Work out the finished part from the listing and answer in its coordinate system (mm). A direction names the side the tool comes from. Give positions to 0.01 mm unless a question says otherwise; leave off trailing zeros. Loops run counter-clockwise (first coordinate to the right, second up) from the corner with the lowest first, then second, coordinate; pieces in that order, holes last.
from build123d import *

# Parameters (mm, degrees)
SKETCH1_W                  = 267
SKETCH1_H                  = 96
BOSS_EXTRUDE1_DEPTH        = 10
SKETCH5_W                  = 261
SKETCH5_H                  = 90
CUT_EXTRUDE2_DEPTH         = 1.7
SKETCH2_R                  = 9.25
CUT_EXTRUDE1_DEPTH         = 10
LPATTERN1_COUNT            = 4
LPATTERN1_PITCH            = 21.5
LPATTERN1_COUNT_DIR2       = 12
LPATTERN1_PITCH_DIR2       = 21.5
ADVANCEDHOLE2_OUTLINE_R    = 2.640558065
ADVANCEDHOLE2_DEPTH        = 7.996
ADVANCEDHOLE2_DRAFT        = -2.3593
ADVANCEDHOLE2_2_OUTLINE_R  = 2.640558065
ADVANCEDHOLE2_2_DEPTH      = 7.996
ADVANCEDHOLE2_2_DRAFT      = -2.3593
ADVANCEDHOLE2_3_OUTLINE_R  = 2.640558065
ADVANCEDHOLE2_3_DEPTH      = 7.996
ADVANCEDHOLE2_3_DRAFT      = -2.3593
ADVANCEDHOLE2_4_OUTLINE_R  = 2.640558065
ADVANCEDHOLE2_4_DEPTH      = 7.996
ADVANCEDHOLE2_4_DRAFT      = -2.3593
ADVANCEDHOLE2_5_OUTLINE_R  = 2.640558065
ADVANCEDHOLE2_5_DEPTH      = 7.996
ADVANCEDHOLE2_5_DRAFT      = -2.3593
ADVANCEDHOLE2_6_OUTLINE_R  = 2.640558065
ADVANCEDHOLE2_6_DEPTH      = 7.996
ADVANCEDHOLE2_6_DRAFT      = -2.3593
ADVANCEDHOLE2_7_OUTLINE_R  = 2.640558065
ADVANCEDHOLE2_7_DEPTH      = 7.996
ADVANCEDHOLE2_7_DRAFT      = -2.3593
ADVANCEDHOLE2_8_OUTLINE_R  = 2.640558065
ADVANCEDHOLE2_8_DEPTH      = 7.996
ADVANCEDHOLE2_8_DRAFT      = -2.3593
ADVANCEDHOLE2_9_OUTLINE_R  = 2.640558065
ADVANCEDHOLE2_9_DEPTH      = 7.996
ADVANCEDHOLE2_9_DRAFT      = -2.3593
ADVANCEDHOLE2_10_OUTLINE_R = 2.640558065
ADVANCEDHOLE2_10_DEPTH     = 7.996
ADVANCEDHOLE2_10_DRAFT     = -2.3593


# Read off the part's stored shape, not the designer's step: AdvancedHole2
with BuildPart() as part:
    # Sketch1 → Boss-Extrude1 (new body)
    with BuildSketch(Plane(origin=(0, 0, 0), x_dir=(1, 0, 0), z_dir=(0, 1, 0))):
        with Locations((133.5, 48)):
            Rectangle(SKETCH1_W, SKETCH1_H)
    extrude(amount=BOSS_EXTRUDE1_DEPTH)

    # Sketch5 → Cut-Extrude2 (cut)
    with BuildSketch(Plane(origin=(0, 10, 0), x_dir=(1, 0, 0), z_dir=(0, 1, 0))):
        with Locations((133.5, 48)):
            Rectangle(SKETCH5_W, SKETCH5_H)
    extrude(amount=-CUT_EXTRUDE2_DEPTH, mode=Mode.SUBTRACT)

    # Sketch2 → Cut-Extrude1 (cut)
    with BuildSketch(Plane(origin=(0, 10, 0), x_dir=(1, 0, 0), z_dir=(0, 1, 0))):
        with Locations(Location((15.25, 15.75, 0), (0, 0, 270))):
            Circle(SKETCH2_R)
    cut_extrude1 = extrude(amount=-CUT_EXTRUDE1_DEPTH, mode=Mode.SUBTRACT)

    # LPattern1: Cut-Extrude1 4 × 12
    with Locations(*[(j * LPATTERN1_PITCH_DIR2, 0, -i * LPATTERN1_PITCH) for i in range(LPATTERN1_COUNT) for j in range(LPATTERN1_COUNT_DIR2) if (i, j) != (0, 0)]):
        add(cut_extrude1, mode=Mode.SUBTRACT)


with BuildPart() as advancedhole2_tool:
    # AdvancedHole2 outline → AdvancedHole2 (with draft: the straight prism first)
    with BuildSketch(Plane(origin=(0, 0.304, 0), x_dir=(1, 0, 0), z_dir=(0, 1, 0))):
        with Locations((155, 69.5)):
            Circle(ADVANCEDHOLE2_OUTLINE_R)
    extrude(amount=ADVANCEDHOLE2_DEPTH)
    # AdvancedHole2: the draft: its side faces are tilted about the plane it starts from
    advancedhole2_sides = [advancedhole2_tool.faces().sort_by_distance(p)[0] for p in [
        (152.359441935, 4.302, -69.5),
    ]]
    draft(advancedhole2_sides, Plane(origin=(0, 0.304, 0), x_dir=(1, 0, 0), z_dir=(0, 1, 0)), ADVANCEDHOLE2_DRAFT)


with BuildPart() as part_1:
    add(part.part)

    # AdvancedHole2: cut by advancedhole2_tool
    add(advancedhole2_tool.part, mode=Mode.SUBTRACT)


with BuildPart() as advancedhole2_2_tool:
    # AdvancedHole2 2 outline → AdvancedHole2 2 (with draft: the straight prism first)
    with BuildSketch(Plane(origin=(0, 0.304, 0), x_dir=(1, 0, 0), z_dir=(0, 1, 0))):
        with Locations((155, 26.5)):
            Circle(ADVANCEDHOLE2_2_OUTLINE_R)
    extrude(amount=ADVANCEDHOLE2_2_DEPTH)
    # AdvancedHole2 2: the draft: its side faces are tilted about the plane it starts from
    advancedhole2_2_sides = [advancedhole2_2_tool.faces().sort_by_distance(p)[0] for p in [
        (152.359441935, 4.302, -26.5),
    ]]
    draft(advancedhole2_2_sides, Plane(origin=(0, 0.304, 0), x_dir=(1, 0, 0), z_dir=(0, 1, 0)), ADVANCEDHOLE2_2_DRAFT)


with BuildPart() as part_2:
    add(part_1.part)

    # AdvancedHole2 2: cut by advancedhole2_2_tool
    add(advancedhole2_2_tool.part, mode=Mode.SUBTRACT)


with BuildPart() as advancedhole2_3_tool:
    # AdvancedHole2 3 outline → AdvancedHole2 3 (with draft: the straight prism first)
    with BuildSketch(Plane(origin=(0, 0.304, 0), x_dir=(1, 0, 0), z_dir=(0, 1, 0))):
        with Locations((112, 26.5)):
            Circle(ADVANCEDHOLE2_3_OUTLINE_R)
    extrude(amount=ADVANCEDHOLE2_3_DEPTH)
    # AdvancedHole2 3: the draft: its side faces are tilted about the plane it starts from
    advancedhole2_3_sides = [advancedhole2_3_tool.faces().sort_by_distance(p)[0] for p in [
        (109.359441935, 4.302, -26.5),
    ]]
    draft(advancedhole2_3_sides, Plane(origin=(0, 0.304, 0), x_dir=(1, 0, 0), z_dir=(0, 1, 0)), ADVANCEDHOLE2_3_DRAFT)


with BuildPart() as part_3:
    add(part_2.part)

    # AdvancedHole2 3: cut by advancedhole2_3_tool
    add(advancedhole2_3_tool.part, mode=Mode.SUBTRACT)


with BuildPart() as advancedhole2_4_tool:
    # AdvancedHole2 4 outline → AdvancedHole2 4 (with draft: the straight prism first)
    with BuildSketch(Plane(origin=(0, 0.304, 0), x_dir=(1, 0, 0), z_dir=(0, 1, 0))):
        with Locations((112, 69.5)):
            Circle(ADVANCEDHOLE2_4_OUTLINE_R)
    extrude(amount=ADVANCEDHOLE2_4_DEPTH)
    # AdvancedHole2 4: the draft: its side faces are tilted about the plane it starts from
    advancedhole2_4_sides = [advancedhole2_4_tool.faces().sort_by_distance(p)[0] for p in [
        (109.359441935, 4.302, -69.5),
    ]]
    draft(advancedhole2_4_sides, Plane(origin=(0, 0.304, 0), x_dir=(1, 0, 0), z_dir=(0, 1, 0)), ADVANCEDHOLE2_4_DRAFT)


with BuildPart() as part_4:
    add(part_3.part)

    # AdvancedHole2 4: cut by advancedhole2_4_tool
    add(advancedhole2_4_tool.part, mode=Mode.SUBTRACT)


with BuildPart() as advancedhole2_5_tool:
    # AdvancedHole2 5 outline → AdvancedHole2 5 (with draft: the straight prism first)
    with BuildSketch(Plane(origin=(0, 0.304, 0), x_dir=(1, 0, 0), z_dir=(0, 1, 0))):
        with Locations((198, 48)):
            Circle(ADVANCEDHOLE2_5_OUTLINE_R)
    extrude(amount=ADVANCEDHOLE2_5_DEPTH)
    # AdvancedHole2 5: the draft: its side faces are tilted about the plane it starts from
    advancedhole2_5_sides = [advancedhole2_5_tool.faces().sort_by_distance(p)[0] for p in [
        (195.359441935, 4.302, -48),
    ]]
    draft(advancedhole2_5_sides, Plane(origin=(0, 0.304, 0), x_dir=(1, 0, 0), z_dir=(0, 1, 0)), ADVANCEDHOLE2_5_DRAFT)


with BuildPart() as part_5:
    add(part_4.part)

    # AdvancedHole2 5: cut by advancedhole2_5_tool
    add(advancedhole2_5_tool.part, mode=Mode.SUBTRACT)


with BuildPart() as advancedhole2_6_tool:
    # AdvancedHole2 6 outline → AdvancedHole2 6 (with draft: the straight prism first)
    with BuildSketch(Plane(origin=(0, 0.304, 0), x_dir=(1, 0, 0), z_dir=(0, 1, 0))):
        with Locations((69, 48)):
            Circle(ADVANCEDHOLE2_6_OUTLINE_R)
    extrude(amount=ADVANCEDHOLE2_6_DEPTH)
    # AdvancedHole2 6: the draft: its side faces are tilted about the plane it starts from
    advancedhole2_6_sides = [advancedhole2_6_tool.faces().sort_by_distance(p)[0] for p in [
        (66.359441935, 4.302, -48),
    ]]
    draft(advancedhole2_6_sides, Plane(origin=(0, 0.304, 0), x_dir=(1, 0, 0), z_dir=(0, 1, 0)), ADVANCEDHOLE2_6_DRAFT)


with BuildPart() as part_6:
    add(part_5.part)

    # AdvancedHole2 6: cut by advancedhole2_6_tool
    add(advancedhole2_6_tool.part, mode=Mode.SUBTRACT)


with BuildPart() as advancedhole2_7_tool:
    # AdvancedHole2 7 outline → AdvancedHole2 7 (with draft: the straight prism first)
    with BuildSketch(Plane(origin=(0, 0.304, 0), x_dir=(1, 0, 0), z_dir=(0, 1, 0))):
        with Locations((26, 26.5)):
            Circle(ADVANCEDHOLE2_7_OUTLINE_R)
    extrude(amount=ADVANCEDHOLE2_7_DEPTH)
    # AdvancedHole2 7: the draft: its side faces are tilted about the plane it starts from
    advancedhole2_7_sides = [advancedhole2_7_tool.faces().sort_by_distance(p)[0] for p in [
        (23.359441935, 4.302, -26.5),
    ]]
    draft(advancedhole2_7_sides, Plane(origin=(0, 0.304, 0), x_dir=(1, 0, 0), z_dir=(0, 1, 0)), ADVANCEDHOLE2_7_DRAFT)


with BuildPart() as part_7:
    add(part_6.part)

    # AdvancedHole2 7: cut by advancedhole2_7_tool
    add(advancedhole2_7_tool.part, mode=Mode.SUBTRACT)


with BuildPart() as advancedhole2_8_tool:
    # AdvancedHole2 8 outline → AdvancedHole2 8 (with draft: the straight prism first)
    with BuildSketch(Plane(origin=(0, 0.304, 0), x_dir=(1, 0, 0), z_dir=(0, 1, 0))):
        with Locations((241, 26.5)):
            Circle(ADVANCEDHOLE2_8_OUTLINE_R)
    extrude(amount=ADVANCEDHOLE2_8_DEPTH)
    # AdvancedHole2 8: the draft: its side faces are tilted about the plane it starts from
    advancedhole2_8_sides = [advancedhole2_8_tool.faces().sort_by_distance(p)[0] for p in [
        (238.359441935, 4.302, -26.5),
    ]]
    draft(advancedhole2_8_sides, Plane(origin=(0, 0.304, 0), x_dir=(1, 0, 0), z_dir=(0, 1, 0)), ADVANCEDHOLE2_8_DRAFT)


with BuildPart() as part_8:
    add(part_7.part)

    # AdvancedHole2 8: cut by advancedhole2_8_tool
    add(advancedhole2_8_tool.part, mode=Mode.SUBTRACT)


with BuildPart() as advancedhole2_9_tool:
    # AdvancedHole2 9 outline → AdvancedHole2 9 (with draft: the straight prism first)
    with BuildSketch(Plane(origin=(0, 0.304, 0), x_dir=(1, 0, 0), z_dir=(0, 1, 0))):
        with Locations((241, 69.5)):
            Circle(ADVANCEDHOLE2_9_OUTLINE_R)
    extrude(amount=ADVANCEDHOLE2_9_DEPTH)
    # AdvancedHole2 9: the draft: its side faces are tilted about the plane it starts from
    advancedhole2_9_sides = [advancedhole2_9_tool.faces().sort_by_distance(p)[0] for p in [
        (238.359441935, 4.302, -69.5),
    ]]
    draft(advancedhole2_9_sides, Plane(origin=(0, 0.304, 0), x_dir=(1, 0, 0), z_dir=(0, 1, 0)), ADVANCEDHOLE2_9_DRAFT)


with BuildPart() as part_9:
    add(part_8.part)

    # AdvancedHole2 9: cut by advancedhole2_9_tool
    add(advancedhole2_9_tool.part, mode=Mode.SUBTRACT)


with BuildPart() as advancedhole2_10_tool:
    # AdvancedHole2 10 outline → AdvancedHole2 10 (with draft: the straight prism first)
    with BuildSketch(Plane(origin=(0, 0.304, 0), x_dir=(1, 0, 0), z_dir=(0, 1, 0))):
        with Locations((26, 69.5)):
            Circle(ADVANCEDHOLE2_10_OUTLINE_R)
    extrude(amount=ADVANCEDHOLE2_10_DEPTH)
    # AdvancedHole2 10: the draft: its side faces are tilted about the plane it starts from
    advancedhole2_10_sides = [advancedhole2_10_tool.faces().sort_by_distance(p)[0] for p in [
        (23.359441935, 4.302, -69.5),
    ]]
    draft(advancedhole2_10_sides, Plane(origin=(0, 0.304, 0), x_dir=(1, 0, 0), z_dir=(0, 1, 0)), ADVANCEDHOLE2_10_DRAFT)


with BuildPart() as part_10:
    add(part_9.part)

    # AdvancedHole2 10: cut by advancedhole2_10_tool
    add(advancedhole2_10_tool.part, mode=Mode.SUBTRACT)


solid = part_10.part
Item 1: Flat-ended cylindrical pins translate along their axes: pin 1 Ø21.5 at (x, z) = (36.75, -58.75) entering from +Y; pin 2 Ø15 at (x, z) = (15.25, -37.25) entering from +Y; pin 3 Ø1.6 at (x, z) = (27, -70.5) entering from +Y. Find the tip coordinate at first contact, or state that the pin passes through.
Item 2: Find section B-B, the plane z = -59.5. Give the number of separate pieces and of enclosed holes in the cut face, plus the area to 3 significant figures.
Item 3: Find section D-D, the plane x = 182.5. Write down the section's boundary in (y, z).
Item 4: Determine the mould class of faces 1 (the face through (132, 5, 0)), 2 (the face through (136.044, 4.208, -54.482)) for opening direction X: released by +X, released by -X, zero draft, split by the parting line, or undercut.
Item 5: Consider line 1 (Z direction, x = 231, y = 6); line 2 (Z direction, x = 199, y = 4.75); line 3 (Z direction, x = 210, y = 4.5). Determine where each line is inside the solid, lowest interval first.
Item 6: For faces 3 (the face through (260.92, 4.21, -81.45)), 4 (the face through (69, 0.304, -48)), determine the directions among +Z, -Z, +X, -X, +Y, -Y from which every point of the face is accessible in a straight line to the end or side of a thin tool.
Item 7: Find section A-A, the plane x = 122.75. Write down the section's boundary in (y, z), plus the area to 3 significant figures.
Ans:
1. pin 1: stops at y = 8.3
1. pin 2: passes through
1. pin 3: stops at y = 0.3
2. separate pieces: 13
2. enclosed holes: 0
2. area: 390 mm2
3. outline: (0, -96) - (10, -96) - (10, -93) - (8.3, -93) - (8.3, -88.19) - (0, -88.19) - close; (0, -72.31) - (8.3, -72.31) - (8.3, -66.69) - (0, -66.69) - close; (0, -50.81) - (8.3, -50.81) - (8.3, -45.19) - (0, -45.19) - close; (0, -29.31) - (8.3, -29.31) - (8.3, -23.69) - (0, -23.69) - close; (0, -7.81) - (8.3, -7.81) - (8.3, -3) - (10, -3) - (10, 0) - (0, 0) - close
4. face 1: zero draft
4. face 2: undercut
5. line 1: z = -96 to -89.47, -71.03 to -67.97, -49.53 to -46.47, -28.03 to -24.97, -6.53 to 0
5. line 2: z = -96 to -50.64, -45.36 to 0
5. line 3: z = -96 to -89.42, -71.08 to -67.92, -49.58 to -46.42, -28.08 to -24.92, -6.58 to 0
6. face 3: +Y, -Y
6. face 4: +Y
7. outline: (0, -96) - (10, -96) - (10, -93) - (8.3, -93) - (8.3, -89.5) - (0, -89.5) - close; (0, -71) - (8.3, -71) - (8.3, -68) - (0, -68) - close; (0, -49.5) - (8.3, -49.5) - (8.3, -46.5) - (0, -46.5) - close; (0, -28) - (8.3, -28) - (8.3, -25) - (0, -25) - close; (0, -6.5) - (8.3, -6.5) - (8.3, -3) - (10, -3) - (10, 0) - (0, 0) - close
7. area: 193 mm2
